Work out the finished part from the listing and answer in its coordinate system (mm). A direction names the side the tool comes from. Round coordinates to 2 decimals unless told otherwise and drop trailing zeros. Loops run counter-clockwise (first coordinate to the right, second up) from the corner with the lowest first, then second, coordinate; pieces in that order, holes last. Notation, with made-up numbers: (-33, 68.25) -> (24, 68.25) arc R16 ccw to (24, 98.25) -> close; hole circle Ø10 at (73.5, 80.25). An arc over 180 degrees is marked (long way). Use one line per item in the form item = value.
```python
from build123d import *

# Parameters (mm, degrees)
SKETCH1_3_W         = 16
SKETCH1_3_H         = 12
BOSS_EXTRUDE2_DEPTH = 8
SKETCH1_4_W         = 16
SKETCH1_4_H         = 8
BOSS_EXTRUDE3_DEPTH = 20


with BuildPart() as part:
    # Sketch1<3> → Boss-Extrude2 (new body)
    with BuildSketch(Plane(origin=(0, 0, 0), x_dir=(1, 0, 0), z_dir=(0, 1, 0))):
        Polygon((-28, 8), (-28, -16), (12, -16), (12, -8), (28, -8), (28, 16), (-12, 16), (-12, 8), align=None)
        Rectangle(SKETCH1_3_W, SKETCH1_3_H, mode=Mode.SUBTRACT)
    extrude(amount=BOSS_EXTRUDE2_DEPTH)

    # Sketch1<4> → Boss-Extrude3 (add)
    with BuildSketch(Plane(origin=(0, 0, 0), x_dir=(1, 0, 0), z_dir=(0, 1, 0))):
        with Locations((20, -12)):
            Rectangle(SKETCH1_4_W, SKETCH1_4_H)
        with Locations((-20, 12)):
            Rectangle(SKETCH1_4_W, SKETCH1_4_H)
    extrude(amount=BOSS_EXTRUDE3_DEPTH)


solid = part.part
```
(1) Find section A-A, the plane y = 16.25. Write down the section's boundary in (x, z), then the cut area to 3 significant figures.
Completed:
outline = (-28, -16) -> (-12, -16) -> (-12, -8) -> (-28, -8) -> close; (12, 8) -> (28, 8) -> (28, 16) -> (12, 16) -> close
area = 256 mm2
(2) Find section B-B, the plane x = -4. Write down the section's boundary in (y, z).
Completed:
outline = (0, -16) -> (8, -16) -> (8, -6) -> (0, -6) -> close; (0, 6) -> (8, 6) -> (8, 16) -> (0, 16) -> close
(3) For faces 4 (the flat face through (-12, 14, -12)), 5 (the flat face through (12, 14, 12)), 6 (the flat face through (0, 4, 6)), determine the directions among +Z, -Z, +X, -X, +Y, -Y from which every point of the face is accessible in a straight line to the end or side of a thin tool.
Completed:
face_4 = +Z, -Z, +X, +Y
face_5 = +Z, -Z, -X, +Y
face_6 = +Y, -Y
(4) Consider L1, parallel to Z at x = 20.5, y = 17.5; L2, parallel to X at y = 2.25, z = 2.5; L3, parallel to Y at x = -8.5, z = -9. Determine where each line is inside the solid, lowest interval first.
Completed:
L1 = 8 to 16
L2 = -28 to -8, 8 to 28
L3 = 0 to 8
(5) For a pull along X with two mould halves and no side action, classify faces 1 (the flat face through (0, 4, -6)), 2 (the flat face through (0, 8, -7)), 3 (the flat face through (-28, 5, -4)) as +X half, -X half, draft (parallel to the pull), parting line (faces both ways), or undercut.
Completed:
face_1 = undercut
face_2 = draft
face_3 = -X half
(6) Find section C-C, the plane y = 6. Write down the section's boundary in (x, z).
Completed:
outline = (-28, -16) -> (28, -16) -> (28, 16) -> (-28, 16) -> close; hole (-8, -6) -> (8, -6) -> (8, 6) -> (-8, 6) -> close
(7) Given P1, Ø4, axis at y = 16, z = 13, coming from the -X side; P2, Ø3, axis at x = 14.5, z = 3.5, coming from the +Y side; P3, Ø4, axis at y = 14.5, z = -10.5, coming from the +X side, each flat-ended and moving along its own axis, determine where each tip first touches the part or whether it passes through.
Completed:
P1 = 12
P2 = 8
P3 = -12
(8) Find section D-D, the plane z = 11. Write down the section's boundary in (x, y).
Completed:
outline = (-28, 0) -> (28, 0) -> (28, 20) -> (12, 20) -> (12, 8) -> (-28, 8) -> close
